Autodesk Inventor part; units mm, degrees
ref_plane "YZ Plane" through (0, 0, 0) normal (1, 0, 0) x (0, 1, 0)
ref_plane "XZ Plane" through (0, 0, 0) normal (0, 1, 0) x (-1, 0, 0)
ref_plane "XY Plane" through (0, 0, 0) normal (0, 0, 1) x (1, 0, 0)
sketch "Sketch1" plane through (0, 0, 0) normal (0, 0, 1) x (1, 0, 0)
  circle A0 centre (0, 0) radius 2.875
  circle A1 centre (0, 0) radius 4.875
  circle A2 centre (0, 0) radius 13.97
  dimension "d0" = 5.75
  dimension "d2" = 2
  dimension "d3" = 27.94
extrude "Extrusion1" add sketch "Sketch1" against normal blind 4.064 contours A1
sketch "Sketch2" plane through (0, 0, 0) normal (0, 0, 1) x (1, 0, 0)
  circle A0 centre (0, 0) radius 4.875
  circle A1 centre (0, 0) radius 1.27
  circle A2 centre (0, 0) radius 13.97
  dimension "d6" = 2.54
  dimension "d7" = 27.94
extrude "Extrusion2" add sketch "Sketch2" along normal mid plane 4 contours A0 | A2
sketch "Sketch3" plane through (0, 0, 0) normal (1, 0, 0) x (0, 1, 0)
  line L0 (13.97, 2) -> (-13.97, 2)
  line L1 (-13.97, -2) -> (13.97, -2)
  line L2 (13.97, 2) -> (13.97, -2)
  circle A0 centre (13.97, 0) radius 1
  line L3 (0, 2) -> (0, -2) construction
  point P0 (0, 0)
  dimension "d10" = 2
revolve "Revolution1" cut sketch "Sketch3" angle 360 about axis through (0, 0, 2) along (0, 0, -1)
sketch "Sketch4" plane through (0, 0, 2) normal (0, 0, 1) x (1, 0, 0)
  circle A0 centre (0, 0) radius 13.97
  line L0 (0, 4.875) -> (0, 13.97)
  line L1 (0, 0) -> (9.9312, 0) construction
  circle A1 centre (-2.0844, -9.8063) radius 1
  arc A2 (0, 4.875) -> (-2.0603, -4.4183) centre (0, 0) ccw
  line L2 (-2.0603, -4.4183) -> (-5.904, -12.6611)
  dimension "d13" = 2
extrude "Extrusion3" cut sketch "Sketch4" against normal blind 4 contours L0 A2 L2 A0 | A1 picked at (-8.1024, 7.2275)
fillet "Fillet1" radius 3.175 2 edges at (0, 4.875, 0) (-2.0603, -4.4183, 0)
properties part number "Pulley"
The model under review builds one solid part; all positions refer to its coordinate system, in mm. A direction names the side the tool comes from. Round coordinates to 2 decimals unless told otherwise and drop trailing zeros. Loops run counter-clockwise (first coordinate to the right, second up) from the corner with the lowest first, then second, coordinate; pieces in that order, holes last. Notation, with made-up numbers: (-30, -16.5) -> (-16, -16.5) arc R27 ccw to (-16, 14.5) -> close; hole circle Ø2 at (62, 52). An arc over 180 degrees is marked (long way). One line per question, with ' | ' between items. Start each with the question number.
Item 1: Add section A-A, the plane y = 0. Write out the cut boundary in (x, z) (3 decimals).
Item 2: Add section B-B, the plane z = -0.5. Write out the cut boundary in (x, y) (3 decimals), then the cut area to 3 significant figures.
Item 3: Machinability: for faces 1 (the face through (0, 11, 0)), 2 (the face through (-0.17, -1.26, -0.03)), 3 (the face through (-0.37, 2.85, -3.02)), which of the approach directions +Z, -Z, +X, -X, +Y, -Y give a long, thin tool a straight path to every point of the face, cutting with its end or side? Answer none if there is none.
Item 4: Wall thickness on line 1 along Y through (x, z) = (0, -3.3) (3 decimals); line 2 along Z through (x, y) = (11.5, -0.5); line 3 along Y through (x, z) = (-4.5, -0.25): over which ranges is each line inside the solid? List them lowest first. Write a range as [from, to].
Item 5: For pin 1 (1 mm diameter, centred on x = 3, z = -3, fed in from -Y); pin 2 (1 mm diameter, centred on x = 6, z = -1.5, fed in from -Y); pin 3 (1 mm diameter, centred on x = 0.5, z = 0, fed in from +Y) (3 decimals), all flat-tipped, find the tip position at first contact; note any pin that passes through.
Item 6: Draft analysis for pull direction Y (two halves, no side actions). For faces 4 (the face through (-0.538, 5.629, 0.028)), 5 (the face through (13.56, -3.36, 1.51)), 6 (the face through (-4.745, 1.118, 0.028)), 7 (the face through (-4.496, -9.641, 0.028)), state which applies: +Y half, -Y half, draft (parallel to the pull), parting line (faces both ways), or undercut.
Return value:
1) outline: (-4.875, -4.064) -> (-2.875, -4.064) -> (-2.875, -2) -> (-1.27, -2) -> (-1.27, 2) -> (-4.875, 2) -> close; (1.27, -2) -> (2.875, -2) -> (2.875, -4.064) -> (4.875, -4.064) -> (4.875, -2) -> (13.97, -2) -> (13.97, -1) arc R1 cw to (13.97, 1) -> (13.97, 2) -> (1.27, 2) -> close
2) outline: (-5.538, -11.876) arc R13.104 ccw (long way) to (0, 13.104) -> (0, 7.397) arc R3.175 cw to (-1.923, 4.48) arc R4.875 ccw to (-3.636, -3.248) arc R3.175 cw to (-3.126, -6.704) -> close; hole circle Ø2 at (-2.084, -9.806); hole circle Ø2.54 at (0, 0) | area: 333 mm2
3) face 1: +Z, -Z, -X, +Y | face 2: +Z, -Z | face 3: -Z
4) line 1: y = [-4.875, -2.875], [2.875, 4.875] | line 2: z = [-2, 2] | line 3: y = [-12.2, -9.65], [-1.88, 1.87]
5) pin 1: stops at y = -4.19 | pin 2: stops at y = -12.84 | pin 3: stops at y = 13.095
6) face 4: +Y half | face 5: parting line | face 6: undercut | face 7: undercut
